Work out the finished part from the listing and answer in its coordinate system (mm). A direction names the side the tool comes from. Give positions to 0.01 mm unless a question says otherwise; leave off trailing zeros. Order: outer loops, then holes, each group sorted by start corner. A loop starts at its lowest first (then second) coordinate and runs counter-clockwise, first axis right, second up.
```python
from build123d import *

# Parameters (mm, degrees)
F0_W      = 114.3
F0_H      = 63.5
F1_DEPTH  = 25.4
F2_W      = 15.875
F2_H      = 63.5
F3_DEPTH  = 11.1125
F4_R      = 9.525
F5_DEPTH  = 25.4
F6_R      = 9.525
F7_DEPTH  = 25.4
F8_W      = 15.875
F8_H      = 63.5
F9_DEPTH  = 19.05
F10_W     = 15.875
F10_H     = 31.75
F11_DEPTH = 19.05
F12_W     = 57.15
F12_H     = 63.5
F12_R     = 9.525
F13_DEPTH = 9.525


with BuildPart() as f1:
    # F0 (on Front) → F1 (new body)
    with BuildSketch(Plane.XZ):
        with Locations((12.284802, -3.837464)):
            Rectangle(F0_W, F0_H)
    extrude(amount=F1_DEPTH)

    # F2 (on face) → F3 (join)
    with BuildSketch(Plane.XZ.offset(25.4)):
        with Locations((-36.927698, -3.837464)):
            Rectangle(F2_W, F2_H)
    extrude(amount=F3_DEPTH)

    # F4 (on face) → F5 (cut)
    with BuildSketch(Plane.XZ.offset(25.4)):
        with Locations((-8.352698, -3.837464)):
            Circle(F4_R)
    extrude(amount=-F5_DEPTH, mode=Mode.SUBTRACT)

    # F6 (on face) → F7 (cut)
    with BuildSketch(Plane.XZ.offset(25.4)):
        with Locations((32.922302, -3.837464)):
            Circle(F6_R)
    extrude(amount=-F7_DEPTH, mode=Mode.SUBTRACT)

    # F8 (on face) → F9 (join)
    with BuildSketch(Plane.XZ.offset(25.4)):
        with Locations((61.497302, -3.837464)):
            Rectangle(F8_W, F8_H)
    extrude(amount=F9_DEPTH)

    # F10 (on face) → F11 (cut)
    with BuildSketch(Plane.XZ.offset(44.45)):
        with Locations((61.497302, -3.837464)):
            Rectangle(F10_W, F10_H)
    extrude(amount=-F11_DEPTH, mode=Mode.SUBTRACT)

    # F12 (on face) → F13 (cut)
    with BuildSketch(Plane(origin=(0, 0, 0), x_dir=(-1, 0, 0), z_dir=(0, 1, 0))):
        with Locations((-40.859802, -3.837464)):
            Rectangle(F12_W, F12_H)
        with Locations((-32.922302, -3.837464)):
            Circle(F12_R, mode=Mode.SUBTRACT)
    extrude(amount=-F13_DEPTH, mode=Mode.SUBTRACT)


solid = f1.part
```
1. The part is cut by section D-D (x = 32). Write down the section's boundary in (y, z) (3 decimals).
Findings below:
outline: (-25.4, -35.587) - (-9.525, -35.587) - (-9.525, -13.318) - (-25.4, -13.318) - close; (-25.4, 5.643) - (-9.525, 5.643) - (-9.525, 27.913) - (-25.4, 27.913) - close
2. Given P1, Ø10.5, axis at y = -4, z = 11, coming from the +X side; P2, Ø6, axis at x = 40, z = 3.5, coming from the -Y side; P3, Ø5.5, axis at y = -33.5, z = -12, coming from the +X side, each flat-ended and moving along its own axis, determine where each tip first touches the part or whether it passes through.
Findings below:
P1: stops at x = 12.28
P2: stops at y = -25.4
P3: stops at x = -28.99
3. Which of the six approach directions +Z, -Z, +X, -X, +Y, -Y give full straight-line access (tool end or side, diameter ignored) to faces 1 (the face through (61, -35, -19.712)), 2 (the face through (53.56, -35, 20)), 3 (the face through (12.285, -5, -4))?
Findings below:
face 1: +X, -Y
face 2: +Z, -Z, -Y
face 3: +Z, -Z, +X, +Y
4. The part is cut by section A-A (y = -31). Write down the section's boundary in (x, z).
Findings below:
outline: (-44.87, -35.59) - (-28.99, -35.59) - (-28.99, 27.91) - (-44.87, 27.91) - close; (53.56, -35.59) - (69.43, -35.59) - (69.43, -19.71) - (53.56, -19.71) - close; (53.56, 12.04) - (69.43, 12.04) - (69.43, 27.91) - (53.56, 27.91) - close
5. The part is cut by section C-C (y = -39.5). Write down the section's boundary in (x, z).
Findings below:
outline: (53.56, -35.59) - (69.43, -35.59) - (69.43, -19.71) - (53.56, -19.71) - close; (53.56, 12.04) - (69.43, 12.04) - (69.43, 27.91) - (53.56, 27.91) - close
6. Straight lines are drawn through the part: probe 1 along Y at (x, z) = (-26, -5); probe 2 along Z at (x, y) = (32.5, -19); probe 3 along Y at (x, z) = (39.5, -28) (3 decimals). For each, find the intervals that lie inside material, in ascending order.
Findings below:
probe 1: y = -25.4 to 0
probe 2: z = -35.59 to -13.35, 5.68 to 27.91
probe 3: y = -25.4 to -9.525
7. The part is cut by section B-B (z = 0.5). Write down the section's boundary in (x, y) (1 decimal), then the cut area to 3 significant figures.
Findings below:
outline: (-44.9, -36.5) - (-29, -36.5) - (-29, -25.4) - (-16.8, -25.4) - (-16.8, 0) - (-44.9, 0) - close; (0.1, -25.4) - (24.4, -25.4) - (24.4, -9.5) - (12.3, -9.5) - (12.3, 0) - (0.1, 0) - close; (41.4, -25.4) - (69.4, -25.4) - (69.4, -9.5) - (41.4, -9.5) - close
area: 1,840 mm2
